```python
from build123d import *
from build123d.topology import SkipClean

# Parameters (mm, degrees)
ESQUISSE1_R             = 2.1
BOSS_EXTRU_1_DEPTH      = 19
ENL_V_START             = -18
ENL_V_MAT_EXTRU_1_DEPTH = 18
ESQUISSE3_R             = 4.5
BOSS_EXTRU_2_DEPTH      = 1.5
ESQUISSE4_R             = 2.5
ENL_V_MAT_EXTRU_2_DEPTH = 2
BOSS_EXTRU_3_DEPTH      = 1


with BuildPart() as part:
    # Esquisse1 → Boss.-Extru.1 (new body)
    with BuildSketch(Plane.XY):
        with BuildLine():
            Line((13.555441712, 3.5), (17.5, 3.5))
            ThreePointArc((17.5, 3.5), (21, 0), (17.5, -3.5))
            Line((17.5, -3.5), (13.555441712, -3.5))
            ThreePointArc((13.555441712, -3.5), (0, -14), (-13.555441712, -3.5))
            Line((-13.555441712, -3.5), (-17.5, -3.5))
            ThreePointArc((-17.5, -3.5), (-21, 0), (-17.5, 3.5))
            Line((-17.5, 3.5), (-13.555441712, 3.5))
            ThreePointArc((-13.555441712, 3.5), (0, 14), (13.555441712, 3.5))
        make_face()
        with Locations((-17.5, 0)):
            Circle(ESQUISSE1_R, mode=Mode.SUBTRACT)
        with Locations((17.5, 0)):
            Circle(ESQUISSE1_R, mode=Mode.SUBTRACT)
    extrude(amount=-BOSS_EXTRU_1_DEPTH)

    # Esquisse2 → Enlèv. mat.-Extru.1 (cut)
    with SkipClean():  # the faces are left unmerged after this step: merging them gives an invalid solid
        with BuildSketch(Plane(origin=(0, 0, -19), x_dir=(-1, 0, 0), z_dir=(0, 0, -1)).offset(ENL_V_START)):
            with BuildLine():
                Line((-13.555441712, 3.5), (-17.5, 3.5))
                ThreePointArc((-17.5, 3.5), (-21, 0), (-17.5, -3.5))
                Line((-17.5, -3.5), (-13.555441712, -3.5))
                ThreePointArc((-13.555441712, -3.5), (-14, 0), (-13.555441712, 3.5))
            make_face()
            with BuildLine():
                Line((13.555441712, 3.5), (17.5, 3.5))
                ThreePointArc((17.5, 3.5), (21, 0), (17.5, -3.5))
                Line((17.5, -3.5), (13.555441712, -3.5))
                ThreePointArc((13.555441712, -3.5), (14, 0), (13.555441712, 3.5))
            make_face()
        extrude(amount=ENL_V_MAT_EXTRU_1_DEPTH, mode=Mode.SUBTRACT)

    # Esquisse3 → Boss.-Extru.2 (add)
    with SkipClean():  # the faces are left unmerged after this step: merging them gives an invalid solid
        with BuildSketch(Plane.XY):
            with Locations((0, 8)):
                Circle(ESQUISSE3_R)
        extrude(amount=BOSS_EXTRU_2_DEPTH)

    # Esquisse4 → Enlèv. mat.-Extru.2 (cut)
    with SkipClean():  # the faces are left unmerged after this step: merging them gives an invalid solid
        with BuildSketch(Plane.XY.offset(1.5)):
            with Locations((0, 8)):
                Circle(ESQUISSE4_R)
        extrude(amount=-ENL_V_MAT_EXTRU_2_DEPTH, mode=Mode.SUBTRACT)

    # Esquisse5 → Boss.-Extru.3 (add)
    with SkipClean():  # the faces are left unmerged after this step: merging them gives an invalid solid
        with BuildSketch(Plane.XY):
            with BuildLine():
                Line((-6.275, -15.975), (6.275, -15.975))
                Line((6.275, -15.975), (6.275, -12.514966041))
                ThreePointArc((6.275, -12.514966041), (0, -14), (-6.275, -12.514966041))
                Line((-6.275, -12.514966041), (-6.275, -15.975))
            make_face()
        extrude(amount=-BOSS_EXTRU_3_DEPTH)


solid = part.part
```
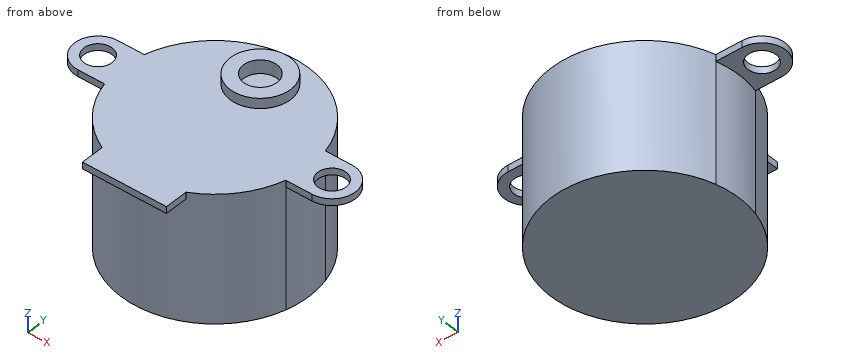
Here's how the part is built. I have some questions about the finished solid (model axes, mm). Coordinates: 2 decimals unless noted, no trailing zeros. Loops run counter-clockwise (first coordinate to the right, second up) from the corner with the lowest first, then second, coordinate; pieces in that order, holes last. Notation, with made-up numbers: (16, -16) - (28, -16) arc R5 ccw to (28, -8) - close; hole circle Ø3 at (43, 78.5). An arc over 180 degrees is marked (long way). Answer as CSV lines item,"result".
Q1. If we section it at D-D, the plane z = -16.75: Write out the boundary of the cut face in (x, y).
Response:
outline,"circle Ø28 at (0, 0)"
Q2. If I drill on L1, parallel to Z at x = 4, y = -5.5; L2, parallel to Z at x = -2, y = 9; L3, parallel to Y at x = -17.5, z = -0.55, over which ranges is the centre line in solid material (lowest first)? Write a range as [from, to].
Response:
L1,"[-19, 0]"
L2,"[-19, -0.5]"
L3,"[-3.5, -2.1], [2.1, 3.5]"
Q3. For pin 1 (12 mm diameter, centred on x = 7, z = -15.5, fed in from +Y); pin 2 (1 mm diameter, centred on y = 0.5, z = -8, fed in from -X); pin 3 (1.1 mm diameter, centred on x = 14.5, z = -0.5, fed in from +Y); pin 4 (5.5 mm diameter, centred on x = 1, y = 8.5, fed in from +Z), each with a flat end and sliding along its axis, tell me the tip position at first contact or that it passes through.
Response:
pin 1,"y = 13.96"
pin 2,"x = -14"
pin 3,"y = 3.5"
pin 4,"z = 1.5"
Q4. If we section it at C-C, the plane x = 0: Write out the boundary of the cut face in (y, z) (3 decimals), and give its area (3 significant figures).
Response:
outline,"(-15.975, -1) - (-14, -1) - (-14, -19) - (14, -19) - (14, 0) - (12.5, 0) - (12.5, 1.5) - (10.5, 1.5) - (10.5, -0.5) - (5.5, -0.5) - (5.5, 1.5) - (3.5, 1.5) - (3.5, 0) - (-15.975, 0) - close"
area,"537 mm2"
Q5. If we section it at A-A, the plane y = 0: Write out the boundary of the cut face in (x, z).
Response:
outline,"(-21, -1) - (-19.6, -1) - (-19.6, 0) - (-21, 0) - close; (-15.4, -1) - (-14, -1) - (-14, -19) - (14, -19) - (14, -1) - (15.4, -1) - (15.4, 0) - (-15.4, 0) - close; (19.6, -1) - (21, -1) - (21, 0) - (19.6, 0) - close"
Q6. If we section it at B-B, the plane x = 17: Write out the boundary of the cut face in (y, z).
Response:
outline,"(-3.5, -1) - (-2.04, -1) - (-2.04, 0) - (-3.5, 0) - close; (2.04, -1) - (3.5, -1) - (3.5, 0) - (2.04, 0) - close"
